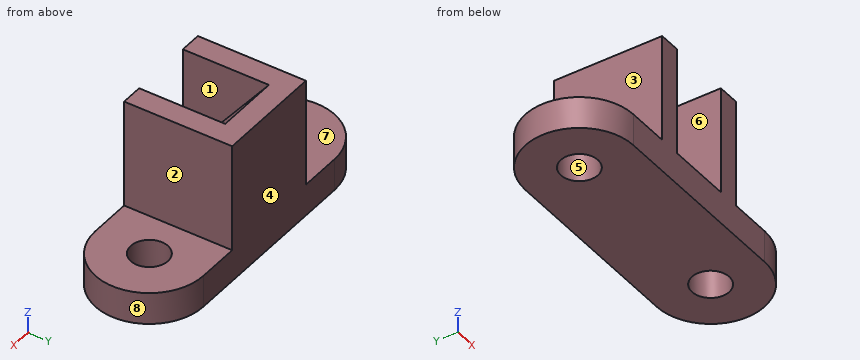
Autodesk Fusion 360 part; units mm, degrees
sketch "Sketch1" plane through (0, 0, 0) normal (0, 0, 1) x (1, 0, 0)
  line L0 (57, 32) -> (-57, 32)
  line L1 (-57, 32) -> (-57, -32)
  line L2 (-57, -32) -> (57, -32)
  line L3 (57, -32) -> (57, 32)
  line L4 (57, 32) -> (-57, -32) construction
  line L5 (-57, 32) -> (57, -32) construction
  circle A0 centre (-57, 0) radius 11
  circle A1 centre (-57, 0) radius 32
  circle A2 centre (57, 0) radius 11
  circle A3 centre (57, 0) radius 32
  dimension "d1" = 114
  dimension "d2" = 64
  dimension "d3" = 22
  dimension "d4" = 32
  dimension "d5" = 22
  dimension "d7" = 32
extrude "Extrude1" add sketch "Sketch1" along normal blind 19 contours L0 L2 A1 A3 | L3 A2 A3 | L3 A2 A3 | L1 A0 A1 | L1 A0 A1
sketch "Sketch2" plane through (0, 0, 19) normal (0, 0, 1) x (-1, 0, 0)
  circle A0 centre (-57, 0) radius 11
  circle A1 centre (57, 0) radius 11
  arc A2 (-57, 32) -> (-57, -32) centre (-57, 0) ccw
  line L0 (-57, -32) -> (57, -32)
  arc A3 (57, -32) -> (57, 32) centre (57, 0) ccw
  line L1 (57, 32) -> (-57, 32)
  line L2 (-32, -32) -> (32, -32)
  line L3 (32, -32) -> (32, 32)
  line L4 (32, 32) -> (-32, 32)
  line L5 (-32, 32) -> (-32, -32)
  line L6 (-32, -32) -> (32, 32) construction
  line L7 (32, -32) -> (-32, 32) construction
  line L8 (19, 32) -> (-19, 32)
  line L9 (-19, 32) -> (-19, -19)
  line L10 (-19, -19) -> (19, -19)
  line L11 (19, -19) -> (19, 32)
  dimension "d10" = 64
  dimension "d11" = 64
  dimension "d12" = 38
  dimension "d13" = 51
  dimension "d14" = 13
  dimension "d15" = 13
extrude "Extrude2" add sketch "Sketch2" along normal blind 64 contours L0 L1 L2 L3 L4 L5 L9 L10 L11
sketch "Sketch3" plane through (19, 0, 0) normal (-1, 0, 0) x (0, -1, 0)
  line L0 (-19, 19) -> (32, 19)
  line L1 (32, 19) -> (32, 83)
  line L2 (32, 83) -> (-19, 83)
  line L3 (-19, 83) -> (-19, 19)
  line L4 (32, 19) -> (-19, 83)
  line L5 (-19, 19) -> (32, 19)
  line L6 (-19, 19) -> (-19, 83)
extrude "Extrude3" add sketch "Sketch3" along normal blind 40 contours L0 L3 L4 L5 L6
equation "d14 = ( ( 64 - 38 ) / 2 ) * 1 mm"
Geometry: final body of the model. Coordinates: model frame, mm. Face numbers are marked on the shaded views. A direction names the side the tool comes from. Give positions to 0.01 mm unless a question says otherwise; leave off trailing zeros. Order: outer loops, then holes, each group sorted by start corner. A loop starts at its lowest first (then second) coordinate and runs counter-clockwise, first axis right, second up. Notation, with made-up numbers: (5, -27) -> (52, -27) arc R13 cw to (52, -7) -> close; hole circle Ø7 at (33, 52.25). An arc over 180 degrees is marked (long way). Answer as a JSON object with one key per item and string values.
Q1. Section B-B (y = -8). Output: boundary loops of the cut face in (x, z), plus the area to 3 significant figures.
Entries:
{"outline": "(-87.98, 0) -> (-64.55, 0) -> (-64.55, 19) -> (-87.98, 19) -> close; (-49.45, 0) -> (49.45, 0) -> (49.45, 19) -> (32, 19) -> (32, 83) -> (19, 83) -> (19, 49.12) -> (-19, 49.12) -> (-19, 83) -> (-32, 83) -> (-32, 19) -> (-49.45, 19) -> close; (64.55, 0) -> (87.98, 0) -> (87.98, 19) -> (64.55, 19) -> close", "area": "5,580 mm^2"}
Q2. Access query for the marked faces 1, 2, 3, 4 and 5. Directions: +Z, -Z, +X, -X, +Y, -Y. A direction counts if a zero-diameter tool reaches every point of the face in a straight line with its end or side. Return the directions, or none.
Entries:
{"face 1": "+Z, -Y", "face 2": "+Z, +X, +Y, -Y", "face 3": "+Z, -X, +Y, -Y", "face 4": "+Z, -Z, +X, -X, +Y", "face 5": "+Z, -Z"}
Q3. Section A-A (x = -64.5). Output: boundary loops of the cut face in (y, z).
Entries:
{"outline": "(-31.11, 0) -> (-8.05, 0) -> (-8.05, 19) -> (-31.11, 19) -> close; (8.05, 0) -> (31.11, 0) -> (31.11, 19) -> (8.05, 19) -> close"}
Q4. Section C-C (z = 23). Output: boundary loops of the cut face in (x, y).
Entries:
{"outline": "(-32, -32) -> (-19, -32) -> (-19, -28.81) -> (19, -28.81) -> (19, -32) -> (32, -32) -> (32, 32) -> (-32, 32) -> close"}
Q5. Draft query along X for the marked faces 6, 7 and 8. Return one class per face: released by +X, released by -X, zero draft, split by the parting line, or undercut.
Entries:
{"face 6": "undercut", "face 7": "zero draft", "face 8": "released by +X"}
Q6. Material intervals for probe 1 along X at (y, z) = (0, 11); probe 2 along Y at (x, z) = (57, 7); probe 3 along X at (y, z) = (3, 79), sorted ascending.
Entries:
{"probe 1": "x = -89 to -68, -46 to 46, 68 to 89", "probe 2": "y = -32 to -11, 11 to 32", "probe 3": "x = -32 to -19, 19 to 32"}
Q7. First-contact query: pin 1 (6 mm diameter, centred on y = 2, z = 72, fed in from -X); pin 2 (17 mm diameter, centred on x = -65, y = -16, fed in from +Z); pin 3 (6 mm diameter, centred on x = -14.5, y = -0.5, fed in from +Z). Flat tips, straight axial feed; report the tip coordinate or a pass-through.
Entries:
{"pin 1": "stops at x = -32", "pin 2": "stops at z = 19", "pin 3": "stops at z = 62.29"}
Q8. Section D-D (y = 26). Output: boundary loops of the cut face in (x, z), plus the area to 3 significant figures.
Entries:
{"outline": "(-75.65, 0) -> (75.65, 0) -> (75.65, 19) -> (32, 19) -> (32, 83) -> (-32, 83) -> (-32, 19) -> (-75.65, 19) -> close", "area": "6,970 mm^2"}
